Autodesk Fusion 360 part; units mm, degrees
sketch "Sketch1" plane through (0, 0, 0) normal (0, 0, 1) x (1, 0, 0)
  line L0 (0, 0) -> (364, 0)
  line L1 (364, 0) -> (364, -230)
  line L2 (364, -230) -> (0, -230)
  line L3 (0, -230) -> (0, 0)
  line L4 (364, -64) -> (0, -64)
extrude "Extrude1" add sketch "Sketch1" along normal blind 6.85 contours L1 L2 L3 L4
extrude "Extrude2" add sketch "Sketch1" along normal blind 11.1 contours L0 L1 L3 L4
sketch "Sketch2" plane through (0, 0, 0) normal (-1, 0, 0) x (0, -1, 0)
  line L0 (0, 0) -> (230, 0)
  line L1 (230, 0) -> (230, 6.85)
  line L2 (230, 6.85) -> (64, 6.85)
  line L3 (64, 6.85) -> (64, 11.1)
  line L4 (64, 11.1) -> (0, 11.1)
  line L5 (0, 11.1) -> (0, 0)
  circle A0 centre (45, 8.1) radius 2
  line L6 (36, 8.5) -> (26, 8.5)
  line L7 (26, 8.5) -> (26, 5.9)
  line L8 (26, 5.9) -> (36, 5.9)
  line L9 (36, 5.9) -> (36, 8.5)
  line L10 (21.4, 9.1) -> (11.4, 9.1)
  line L11 (11.4, 9.1) -> (11.4, 5.45)
  line L12 (11.4, 5.45) -> (21.4, 5.45)
  line L13 (21.4, 5.45) -> (21.4, 9.1)
  dimension "d10" = 4
extrude "Extrude3" add sketch "Sketch2" along normal blind 0.5 contours A0
extrude "Extrude4" cut sketch "Sketch2" against normal blind 9 contours L6 L7 L8 L9 | L10 L11 L12 L13
sketch "Sketch3" plane through (0, 0, 5.9) normal (0, 0, 1) x (-1, 0, 0)
  line L0 (0, 26) -> (0, 36)
  line L1 (0, 36) -> (-9, 36)
  line L2 (-9, 36) -> (-9, 26)
  line L3 (-9, 26) -> (0, 26)
  circle A0 centre (-4, 31) radius 4.5
extrude "Extrude5" add sketch "Sketch3" along normal blind 2.6 contours L0 A0 | L0 A0
sketch "Sketch4" plane through (364, 0, 0) normal (1, 0, 0) x (0, 1, 0)
  line L0 (-230, 0) -> (0, 0)
  line L1 (0, 0) -> (0, 11.1)
  line L2 (0, 11.1) -> (-64, 11.1)
  line L3 (-64, 11.1) -> (-64, 6.85)
  line L4 (-64, 6.85) -> (-230, 6.85)
  line L5 (-230, 6.85) -> (-230, 0)
  line L6 (-21, 8.8) -> (-31, 8.8)
  line L7 (-31, 8.8) -> (-31, 5.15)
  line L8 (-31, 5.15) -> (-21, 5.15)
  line L9 (-21, 5.15) -> (-21, 8.8)
  line L10 (-39.5, 9.4) -> (-51, 9.4)
  line L11 (-51, 9.4) -> (-51, 6.9)
  line L12 (-51, 6.9) -> (-39.5, 6.9)
  line L13 (-39.5, 6.9) -> (-39.5, 9.4)
extrude "Extrude6" cut sketch "Sketch4" against normal blind 10 contours L6 L7 L8 L9 | L10 L11 L12 L13
Could you check a few things on this model? Use its own coordinates, in mm. A direction names the side the tool comes from. Give positions to 0.01 mm unless a question says otherwise; leave off trailing zeros. Loops run counter-clockwise (first coordinate to the right, second up) from the corner with the lowest first, then second, coordinate; pieces in that order, holes last. Notation, with made-up numbers: (73, -20.75) - (97, -20.75) arc R10 ccw to (97, -8.75) - close; hole circle Ø4 at (17, 70). An arc over 180 degrees is marked (long way). Answer in a Markdown table with one row per item. Add a question column.
Q1. For pin 1 (3 mm diameter, centred on x = 6.5, z = 7.5, fed in from +Y); pin 2 (2 mm diameter, centred on y = -128, z = 2, fed in from -X); pin 3 (0.8 mm diameter, centred on x = 6.5, z = 7.5, fed in from -Y), each with a flat end and sliding along its axis, tell me the tip position at first contact or that it passes through.
Q2. If we section it at B-B (y = -75): List the corners of the cut face in (x, z) for me.
Q3. If we section it at A-A (x = 4): List the corners of the cut face in (y, z) for me, plus the area to 3 significant figures.
Q4. Which directions (+Z, -Z, +X, -X, +Y, -Y) give clear straight access to the entire face, cutting with the end or side of a thin tool? Please do faces 5 (the face through (179, -32, 11.1)), 6 (the face through (179, -113, 0)), 7 (the face through (359, -26, 8.8)), 8 (the face through (4, -16, 5.45)), 9 (the face through (8.8, -31, 8.5)).
Q5. Please list where these lines run through material, in increasing order: L1, parallel to Y at x = 173, z = 9; L2, parallel to Z at x = 66.5, y = -153.5; L3, parallel to X at y = -91.5, z = 1.5. Write a range as from..to.
Q6. If we section it at C-C (x = 91): List the corners of the cut face in (y, z) for me.
Q7. We'd pull the mould along Y, two halves only. Please class faces 1 (the face through (185, -230, 3)), 2 (the face through (179, 0, 5)), 3 (the face through (179, -146, 6.85)), 4 (the face through (359, -45, 6.9)): +Y half, -Y half, draft (parallel to the pull), parting line (faces both ways), or undercut.
The answers:
| question | item | result |
|---|---|---|
| 1 | pin 1 | stops at y = 0 |
| 1 | pin 2 | stops at x = 0 |
| 1 | pin 3 | stops at y = -64 |
| 2 | outline | (0, 0) - (364, 0) - (364, 6.85) - (0, 6.85) - close |
| 3 | outline | (-230, 0) - (0, 0) - (0, 11.1) - (-64, 11.1) - (-64, 6.85) - (-230, 6.85) - close; hole (-36, 5.9) - (-35.5, 5.9) - (-35.5, 8.5) - (-36, 8.5) - close; hole (-26.5, 5.9) - (-26, 5.9) - (-26, 8.5) - (-26.5, 8.5) - close; hole (-21.4, 5.45) - (-11.4, 5.45) - (-11.4, 9.1) - (-21.4, 9.1) - close |
| 3 | area | 1,810 mm^2 |
| 4 | face 5 | +Z, +X, -X, +Y, -Y |
| 4 | face 6 | -Z, +X, -X, +Y, -Y |
| 4 | face 7 | +X |
| 4 | face 8 | -X |
| 4 | face 9 | none |
| 5 | L1 | y = -64..0 |
| 5 | L2 | z = 0..6.85 |
| 5 | L3 | x = 0..364 |
| 6 | outline | (-230, 0) - (0, 0) - (0, 11.1) - (-64, 11.1) - (-64, 6.85) - (-230, 6.85) - close |
| 7 | face 1 | -Y half |
| 7 | face 2 | +Y half |
| 7 | face 3 | draft |
| 7 | face 4 | undercut |
